Build history of the part. All positions in model axes, mm. A direction names the side the tool comes from. Coordinates: 2 decimals unless noted, no trailing zeros. Loops run counter-clockwise (first coordinate to the right, second up) from the corner with the lowest first, then second, coordinate; pieces in that order, holes last. Notation, with made-up numbers: (-26, 65.25) - (-3, 65.25) arc R25 cw to (-3, 78.25) - close; hole circle Ø6 at (29.5, 24.25). An arc over 180 degrees is marked (long way). One line per item, written item: value.
Autodesk Inventor part; units mm, degrees
ref_plane "YZ Plane" through (0, 0, 0) normal (1, 0, 0) x (0, 1, 0)
ref_plane "XZ Plane" through (0, 0, 0) normal (0, 1, 0) x (-1, 0, 0)
ref_plane "XY Plane" through (0, 0, 0) normal (0, 0, 1) x (1, 0, 0)
sketch "Sketch1" plane through (0, 0, 0) normal (0, 0, 1) x (1, 0, 0)
  line L0 (-25.6928, -3.3339) -> (25.3072, -3.3339)
  line L1 (25.3072, -3.3339) -> (25.3072, -5.3339)
  line L2 (25.3072, -5.3339) -> (-25.6928, -5.3339)
  line L3 (-25.6928, -5.3339) -> (-25.6928, -3.3339)
  line L4 (-25.6928, -5.3339) -> (-22.6928, -5.3339)
  line L5 (-22.6928, -5.3339) -> (-22.6928, 2.1661)
  line L6 (-22.6928, 2.1661) -> (-25.6928, 2.1661)
  line L7 (-25.6928, 2.1661) -> (-25.6928, -5.3339)
  line L8 (-25.6928, 2.1661) -> (-19.6928, 2.1661)
  line L9 (-19.6928, 2.1661) -> (-19.6928, 0.1661)
  line L10 (-19.6928, 0.1661) -> (-25.6928, 0.1661)
  line L11 (-25.6928, 0.1661) -> (-25.6928, 2.1661)
  line L12 (25.3072, -5.3339) -> (22.3072, -5.3339)
  line L13 (22.3072, -5.3339) -> (22.3072, 2.1661)
  line L14 (22.3072, 2.1661) -> (25.3072, 2.1661)
  line L15 (25.3072, 2.1661) -> (25.3072, -5.3339)
  line L16 (25.3072, 2.1661) -> (19.3072, 2.1661)
  line L17 (19.3072, 2.1661) -> (19.3072, 0.1661)
  line L18 (19.3072, 0.1661) -> (25.3072, 0.1661)
  line L19 (25.3072, 0.1661) -> (25.3072, 2.1661)
  point P0 (0, 0)
  dimension "d0" = 45
  dimension "d1" = 3.5
  dimension "d2" = 6
  dimension "d3" = 6
  dimension "d4" = 51
  dimension "d5" = 3
  dimension "d6" = 2
  dimension "d7" = 3
  dimension "d8" = 2
  dimension "d9" = 2
extrude "Extrusion1" add sketch "Sketch1" along normal blind 10
properties part number "Side Grapper"
Item 1: Cut at D-D, the plane x = 14.5. Write the cut outline in (y, z).
Check result:
outline: (-5.33, 0) - (-3.33, 0) - (-3.33, 10) - (-5.33, 10) - close
Item 2: Cut at A-A, the plane y = 1. Write the cut outline in (x, z), then the cut area to 3 significant figures.
Check result:
outline: (-25.69, 0) - (-19.69, 0) - (-19.69, 10) - (-25.69, 10) - close; (19.31, 0) - (25.31, 0) - (25.31, 10) - (19.31, 10) - close
area: 120 mm^2
Item 3: Tool access for faces 1 (the face through (21, 0.166, 5)), 2 (the face through (-23, 2.166, 5)), 3 (the face through (-19.693, 1, 5)): list every direction of +Z, -Z, +X, -X, +Y, -Y with a clear straight run to the whole face (end or side of a thin tool).
Check result:
face 1: +Z, -Z
face 2: +Z, -Z, +X, -X, +Y
face 3: +Z, -Z, +Y
Item 4: Cut at B-B, the plane z = 8. Write the cut outline in (x, y).
Check result:
outline: (-25.69, -5.33) - (25.31, -5.33) - (25.31, 2.17) - (19.31, 2.17) - (19.31, 0.17) - (22.31, 0.17) - (22.31, -3.33) - (-22.69, -3.33) - (-22.69, 0.17) - (-19.69, 0.17) - (-19.69, 2.17) - (-25.69, 2.17) - close
Item 5: Cut at C-C, the plane y = -1. Write the cut outline in (x, z), then the cut area to 3 significant figures.
Check result:
outline: (-25.69, 0) - (-22.69, 0) - (-22.69, 10) - (-25.69, 10) - close; (22.31, 0) - (25.31, 0) - (25.31, 10) - (22.31, 10) - close
area: 60.0 mm^2
Item 6: Drop flat-ended pins along their axis: P1, Ø3, axis at x = -19, y = -1.5, coming from the -Z side; P2, Ø3, axis at x = -5, z = 2.5, coming from the +Y side. Give the stop position or say it passes through.
Check result:
P1: passes through
P2: stops at y = -3.33
Item 7: Probe probe 1 along X at (y, z) = (-1.75, 3.25); probe 2 along Y at (x, z) = (-20, 5.75); probe 3 along X at (y, z) = (1.75, 5.75). List the from-to ranges inside material, lowest first. Write a range as from..to.
Check result:
probe 1: x = -25.69..-22.69, 22.31..25.31
probe 2: y = -5.33..-3.33, 0.17..2.17
probe 3: x = -25.69..-19.69, 19.31..25.31
Item 8: Pull direction Y, two halves, no side cores. Call faces 4 (the face through (-21, 0.166, 5)), 5 (the face through (0, -4, 0)), 6 (the face through (22.307, -2, 5)), 7 (the face through (22, 2.166, 5)): released by +Y, released by -Y, zero draft, split by the parting line, or undercut.
Check result:
face 4: undercut
face 5: zero draft
face 6: undercut
face 7: released by +Y
